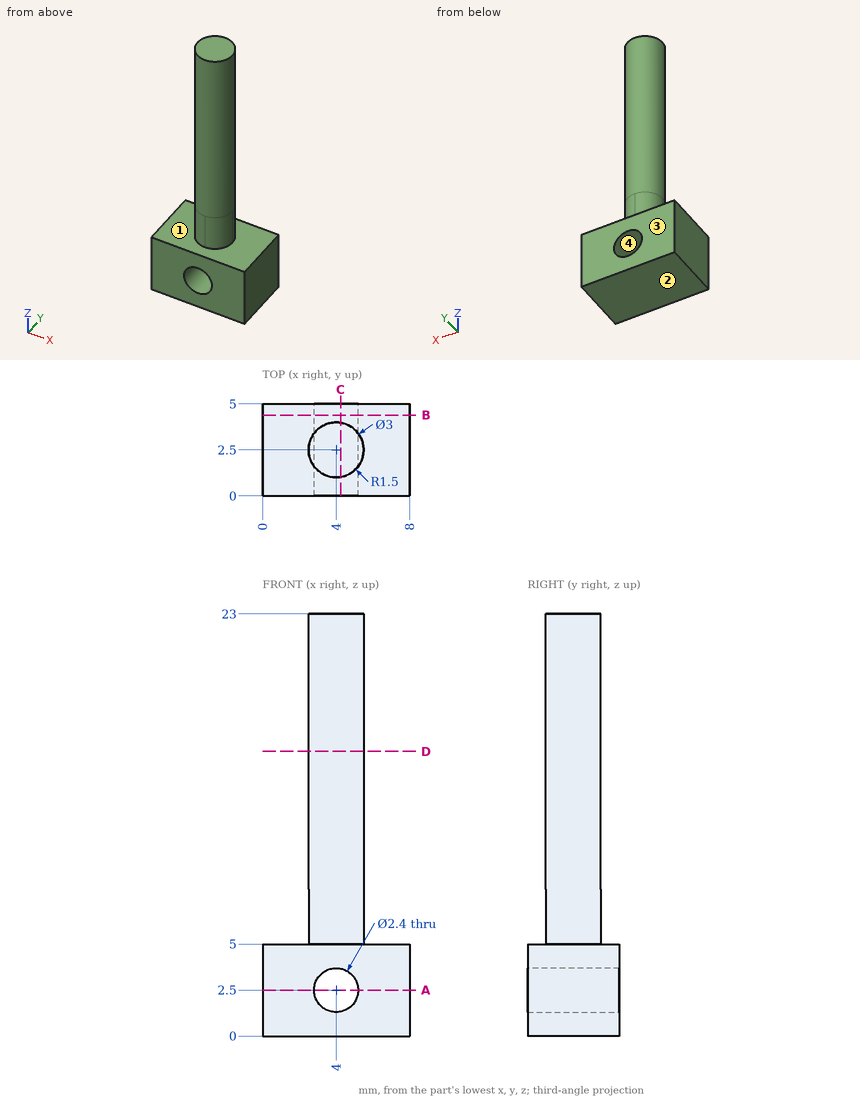
The figure shows three views and two pictorial views of one solid part (mm, origin at its lowest corner). Answer the questions. Coordinates: 2 decimals unless noted, no trailing zeros. Write each loop counter-clockwise with the first axis right and the second up, starting at its lowest first coordinate (ties: lowest second). Pieces come first, ordered by that corner, then holes.
1. The part is cut by section C-C, the plane x = 4.25. Write down the section's boundary in (y, z).
Results list:
outline: (0, 0) - (5, 0) - (5, 1.33) - (0, 1.33) - close; (0, 3.67) - (5, 3.67) - (5, 5) - (3.98, 5) - (3.98, 23) - (1.02, 23) - (1.02, 5) - (0, 5) - close
2. The part is cut by section D-D, the plane z = 15.5. Write down the section's boundary in (x, y), and give its area (3 significant figures).
Results list:
outline: circle Ø3 at (4, 2.5)
area: 7.07 mm2
3. A flat-ended cylindrical pin translates along its axis: pin 1 (1.4 mm diameter, centred on x = 4, z = 2.5, fed in from -Y) (3 decimals). Find the tip coordinate at first contact, or state that the pin passes through.
Results list:
pin 1: passes through
4. The part is cut by section B-B, the plane y = 4.4. Write down the section's boundary in (x, z), and give its area (3 significant figures).
Results list:
outline: (0, 0) - (8, 0) - (8, 5) - (0, 5) - close; hole circle Ø2.4 at (4, 2.5)
area: 35.5 mm2
5. The part is cut by section A-A, the plane z = 2.5. Write down the section's boundary in (x, y), and give its area (3 significant figures).
Results list:
outline: (0, 0) - (2.8, 0) - (2.8, 5) - (0, 5) - close; (5.2, 0) - (8, 0) - (8, 5) - (5.2, 5) - close
area: 28.0 mm2
6. For a pull along Z with two mould halves and no side action, classify the marked faces 1, 2, 3 and 4 as +Z half, -Z half, draft (parallel to the pull), parting line (faces both ways), or undercut.
Results list:
face 1: +Z half
face 2: -Z half
face 3: draft
face 4: undercut
7. Consider line 1 along X through (y, z) = (2.75, 2.5); line 2 along X through (y, z) = (2.5, 17.25); line 3 along X through (y, z) = (3.4, 13.75). Determine where each line is inside the solid, lowest interval first.
Results list:
line 1: x = 0 to 2.8, 5.2 to 8
line 2: x = 2.5 to 5.5
line 3: x = 2.8 to 5.2
